Study the drawing (mm; zero at the part's minimum x, y, z) and answer. Round coordinates to 2 decimals unless told otherwise and drop trailing zeros. Loops run counter-clockwise (first coordinate to the right, second up) from the corner with the lowest first, then second, coordinate; pieces in that order, holes last. Notation, with made-up numbers: (46, 49.25) - (77, 49.25) arc R24 cw to (77, 76.25) - close; hole circle Ø2 at (20.25, 36). An arc over 180 degrees is marked (long way). One line per item, written item: value.
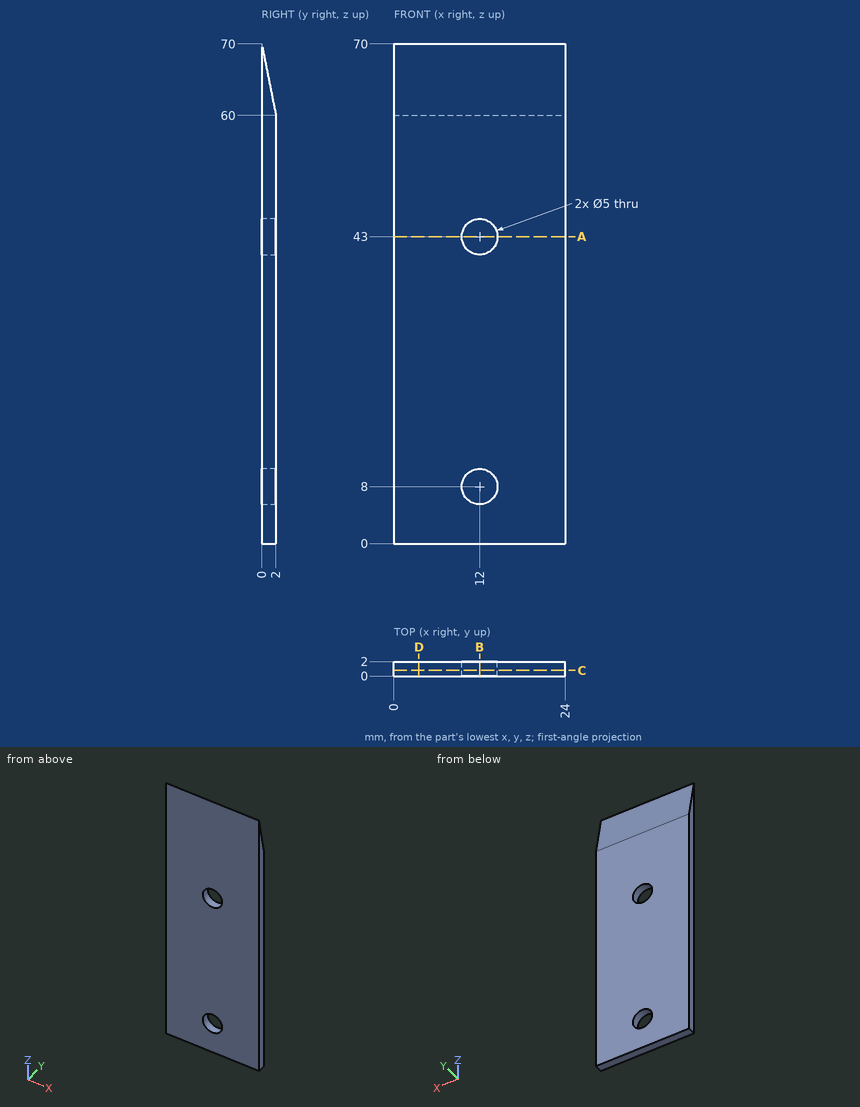
1) A cutting plane is placed at C-C on y = 0.8. Give the vertices of the cut face in (x, z).
Final values:
outline: (0, 0) - (24, 0) - (24, 66) - (0, 66) - close; hole circle Ø5 at (12, 8); hole circle Ø5 at (12, 43)
2) A cutting plane is placed at B-B on x = 12. Give the vertices of the cut face in (y, z), and give its area (3 significant figures).
Final values:
outline: (0, 0) - (2, 0) - (2, 5.5) - (0, 5.5) - close; (0, 10.5) - (2, 10.5) - (2, 40.5) - (0, 40.5) - close; (0, 45.5) - (2, 45.5) - (2, 60) - (0, 70) - close
area: 110 mm2
3) A cutting plane is placed at D-D on x = 3.5. Give the vertices of the cut face in (y, z), and give its area (3 significant figures).
Final values:
outline: (0, 0) - (2, 0) - (2, 60) - (0, 70) - close
area: 130 mm2
4) Consider L1, parallel to X at y = 1.5, z = 8; L2, parallel to X at y = 0.7, z = 6.5. Determine where each line is inside the solid, lowest interval first.
Final values:
L1: 0 to 9.5, 14.5 to 24
L2: 0 to 10, 14 to 24
5) A cutting plane is placed at A-A on z = 43. Give the vertices of the cut face in (x, y).
Final values:
outline: (0, 0) - (9.5, 0) - (9.5, 2) - (0, 2) - close; (14.5, 0) - (24, 0) - (24, 2) - (14.5, 2) - close
